The listing builds one solid part. Answer for the finished solid, in the listing's coordinates (mm). Coordinates: 2 decimals unless noted, no trailing zeros. Loops run counter-clockwise (first coordinate to the right, second up) from the corner with the lowest first, then second, coordinate; pieces in that order, holes last. Notation, with made-up numbers: (67, 6.5) - (94, 6.5) arc R34 cw to (94, 44.5) - close; hole circle Ø7 at (18.5, -18.75). An arc over 180 degrees is marked (long way). Put each result on its own line as item: value.
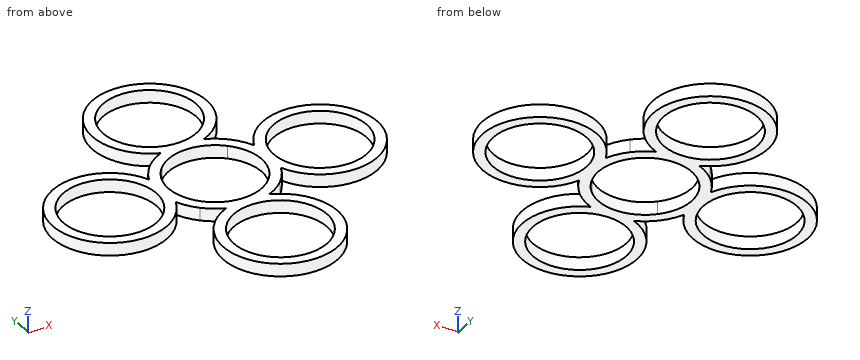
```python
from build123d import *

# Parameters (mm, degrees)
F0_R     = 11
F1_DEPTH = 3


with BuildPart() as f1:
    # F0 (on Top) → F1 (new body)
    with BuildSketch(Plane.XY):
        with BuildLine():
            ThreePointArc((5.09902, 12.5), (0, 38.5), (-5.09902, 12.5))
            ThreePointArc((-5.09902, 12.5), (-7.469962, 11.244984), (-9.545942, 9.545942))
            ThreePointArc((-9.545942, 9.545942), (-11.244984, 7.469962), (-12.5, 5.09902))
            ThreePointArc((-12.5, 5.09902), (-38.5, 0), (-12.5, -5.09902))
            ThreePointArc((-12.5, -5.09902), (-11.244984, -7.469962), (-9.545942, -9.545942))
            ThreePointArc((-9.545942, -9.545942), (-7.469962, -11.244984), (-5.09902, -12.5))
            ThreePointArc((-5.09902, -12.5), (0, -38.5), (5.09902, -12.5))
            ThreePointArc((5.09902, -12.5), (7.469962, -11.244984), (9.545942, -9.545942))
            ThreePointArc((9.545942, -9.545942), (11.244984, -7.469962), (12.5, -5.09902))
            ThreePointArc((12.5, -5.09902), (38.5, 0), (12.5, 5.09902))
            ThreePointArc((12.5, 5.09902), (11.244984, 7.469962), (9.545942, 9.545942))
            ThreePointArc((9.545942, 9.545942), (7.469962, 11.244984), (5.09902, 12.5))
        make_face()
        with Locations((0, -25)):
            Circle(F0_R, mode=Mode.SUBTRACT)
        with Locations((-25, 0)):
            Circle(F0_R, mode=Mode.SUBTRACT)
        with BuildLine():
            ThreePointArc((-7.778175, 7.778175), (0, 11), (7.778175, 7.778175))
            ThreePointArc((7.778175, 7.778175), (11, 0), (7.778175, -7.778175))
            ThreePointArc((7.778175, -7.778175), (0, -11), (-7.778175, -7.778175))
            ThreePointArc((-7.778175, -7.778175), (-11, 0), (-7.778175, 7.778175))
        make_face(mode=Mode.SUBTRACT)
        with Locations((25, 0)):
            Circle(F0_R, mode=Mode.SUBTRACT)
        with Locations((0, 25)):
            Circle(F0_R, mode=Mode.SUBTRACT)
    extrude(amount=F1_DEPTH)


solid = f1.part
```
1) The part is cut by section A-A (y = -25). Give the vertices of the cut face in (x, z).
Found:
outline: (-13.5, 0) - (-11, 0) - (-11, 3) - (-13.5, 3) - close; (11, 0) - (13.5, 0) - (13.5, 3) - (11, 3) - close
2) The part is cut by section C-C (z = 2.5). Give the vertices of the cut face in (x, y).
Found:
outline: (-12.5, -5.1) arc R13.5 ccw to (-9.55, -9.55) arc R13.5 ccw to (-5.1, -12.5) arc R13.5 ccw (long way) to (5.1, -12.5) arc R13.5 ccw to (9.55, -9.55) arc R13.5 ccw to (12.5, -5.1) arc R13.5 ccw (long way) to (12.5, 5.1) arc R13.5 ccw to (9.55, 9.55) arc R13.5 ccw to (5.1, 12.5) arc R13.5 ccw (long way) to (-5.1, 12.5) arc R13.5 ccw to (-9.55, 9.55) arc R13.5 ccw to (-12.5, 5.1) arc R13.5 ccw (long way) to start; hole circle Ø22 at (-25, 0); hole circle Ø22 at (0, -25); hole circle Ø22 at (0, 25); hole (-7.78, -7.78) arc R11 ccw to (7.78, -7.78) arc R11 ccw to (7.78, 7.78) arc R11 ccw to (-7.78, 7.78) arc R11 ccw to start; hole circle Ø22 at (25, 0)
3) The part is cut by section D-D (y = 6). Give the vertices of the cut face in (x, z), and give its area (3 significant figures).
Found:
outline: (-37.09, 0) - (-34.22, 0) - (-34.22, 3) - (-37.09, 3) - close; (-15.78, 0) - (-12.91, 0) - (-12.91, 3) - (-15.78, 3) - close; (-12.09, 0) - (-9.22, 0) - (-9.22, 3) - (-12.09, 3) - close; (9.22, 0) - (12.09, 0) - (12.09, 3) - (9.22, 3) - close; (12.91, 0) - (15.78, 0) - (15.78, 3) - (12.91, 3) - close; (34.22, 0) - (37.09, 0) - (37.09, 3) - (34.22, 3) - close
area: 51.7 mm^2
4) Straight lines are drawn through the part: L1, parallel to Y at x = 6.5, z = 2.7; L2, parallel to X at y = 4.5, z = 1.45; L3, parallel to Y at x = -7, z = 1. For each, find the intervals that lie inside material, in ascending order. Write a range as [from, to].
Found:
L1: y = [-36.83, -33.87], [-16.13, -13.17], [-11.83, -8.87], [8.87, 11.83], [13.17, 16.13], [33.87, 36.83]
L2: x = [-37.73, -35.04], [-14.96, -10.04], [10.04, 14.96], [35.04, 37.73]
L3: y = [-36.54, -33.49], [-16.51, -13.46], [-11.54, -8.49], [8.49, 11.54], [13.46, 16.51], [33.49, 36.54]
5) This flat-tipped pin is pushed along its axis until it touches: pin 1 (20 mm diameter, centred on x = 25, y = 0, fed in from +Z). Where does it stop, or does it pass through?
Found:
pin 1: passes through
